The listing builds one solid part. Answer for the finished solid, in the listing's coordinates (mm). A direction names the side the tool comes from. Coordinates: 2 decimals unless noted, no trailing zeros. Write each loop counter-clockwise with the first axis right and the second up, starting at its lowest first coordinate (ties: lowest second). Pieces come first, ordered by that corner, then holes. Notation, with made-up numbers: M -28,52 L -18,52 A27 cw -18,73 Z; hole C -6,-7 d7. An arc over 180 degrees is marked long. Put each result on its own line as item: value. Start each with the question number.
```python
from build123d import *

# Parameters (mm, degrees)
BOSS_EXTRUDE1_DEPTH       = 25.4
F_4_0MM_DOWEL_HOLE1_D     = 4
F_4_0MM_DOWEL_HOLE1_DEPTH = 3.175
CUT_EXTRUDE1_REACH        = 51.202
SKETCH7_R                 = 5.08
SKETCH7_R_2               = 1.143
FILLET1_R                 = 3.175


with BuildPart() as part:
    # Sketch1 → Boss-Extrude1 (new body)
    with BuildSketch(Plane.XY):
        Polygon((-17.059275079, -16.268900152), (-29.759275079, -16.268900152), (-29.759275079, -36.588900152), (36.915724921, -36.588900152), (36.915724921, -33.413900152), (-26.584275079, -33.413900152), (-26.584275079, -19.443900152), (-17.059275079, -19.443900152), align=None)
    extrude(amount=BOSS_EXTRUDE1_DEPTH)

    # Ø4.0mm Dowel Hole1
    with Locations(Plane(origin=(0, -16.268900152, 0), x_dir=(1, 0, 0), z_dir=(0, 1, 0))):
        with Locations((-21.821775079, -7.9375), (-21.821775079, -17.4625)):
            Hole(F_4_0MM_DOWEL_HOLE1_D / 2, depth=F_4_0MM_DOWEL_HOLE1_DEPTH)

    # Sketch7 → Cut-Extrude1 (cut, up to next)
    with BuildSketch(Plane.XZ.offset(36.588900152), mode=Mode.PRIVATE) as cut_extrude1_sk1:
        with Locations(Location((23.199724921, 12.7, 0), (0, 0, 270))):
            Circle(SKETCH7_R)
    cut_extrude1_tool1 = extrude(cut_extrude1_sk1.sketch, amount=-CUT_EXTRUDE1_REACH, mode=Mode.PRIVATE) & part.part
    # Sketch7 → Cut-Extrude1 (cut, up to next)
    with BuildSketch(Plane.XZ.offset(36.588900152), mode=Mode.PRIVATE) as cut_extrude1_sk2:
        with Locations(Location((23.199724921, 5.2578, 0), (0, 0, 270))):
            Circle(SKETCH7_R_2)
    cut_extrude1_tool2 = extrude(cut_extrude1_sk2.sketch, amount=-CUT_EXTRUDE1_REACH, mode=Mode.PRIVATE) & part.part
    # Sketch7 → Cut-Extrude1 (cut, up to next)
    with BuildSketch(Plane.XZ.offset(36.588900152), mode=Mode.PRIVATE) as cut_extrude1_sk3:
        with Locations(Location((23.199724921, 20.1422, 0), (0, 0, 270))):
            Circle(SKETCH7_R_2)
    cut_extrude1_tool3 = extrude(cut_extrude1_sk3.sketch, amount=-CUT_EXTRUDE1_REACH, mode=Mode.PRIVATE) & part.part
    add(cut_extrude1_tool1.solids().sort_by_distance((23.199725, -36.5889, 12.7))[0], mode=Mode.SUBTRACT)
    add(cut_extrude1_tool2.solids().sort_by_distance((23.199725, -36.5889, 5.2578))[0], mode=Mode.SUBTRACT)
    add(cut_extrude1_tool3.solids().sort_by_distance((23.199725, -36.5889, 20.1422))[0], mode=Mode.SUBTRACT)

    # Fillet1
    fillet1_edges = [part.edges().sort_by_distance(p)[0] for p in [
        (-26.584275079, -33.413900152, 12.7),
        (-29.759275079, -36.588900152, 12.7),
        (-29.759275079, -16.268900152, 12.7),
    ]]
    fillet(fillet1_edges, radius=FILLET1_R)


solid = part.part
```
1) Straight lines are drawn through the part: probe 1 along Y at (x, z) = (-19.5, 9.25); probe 2 along Y at (x, z) = (-7, 9.25); probe 3 along Z at (x, y) = (-21, -18.25). For each, find the intervals that lie inside material, in ascending order.
2) For faces 4 (the face through (-26.584, -25, 13)), 5 (the face through (-17.059, -18, 13)), 6 (the face through (-20.235, -17.879, 18.679)), determine the directions among +Z, -Z, +X, -X, +Y, -Y from which every point of the face is accessible in a straight line to the end or side of a thin tool.
3) A cutting plane is placed at C-C on x = 2.5. Write down the section's boundary in (y, z), then the cut area to 3 significant figures.
4) Given pin 1 Ø10 at (y, z) = (-26.5, 14) entering from +X; pin 2 Ø1.5 at (y, z) = (-19, 5.5) entering from +X; pin 3 Ø5.5 at (y, z) = (-26.5, 17) entering from +X, each flat-ended and moving along its own axis, determine where each tip first touches the part or whether it passes through.
5) A cutting plane is placed at A-A on z = 12.7. Write down the section's boundary in (x, y) (3 decimals).
6) A cutting plane is placed at D-D on y = -24.5. Write down the section's boundary in (x, z), then the cut area to 3 significant figures.
7) A cutting plane is placed at B-B on z = 20.5. Write down the section's boundary in (x, y) (3 decimals), then the cut area to 3 significant figures.
8) Determine the mould class of faces 1 (the face through (-4, -34, 0)), 2 (the face through (24.333, -35.024, 5.407)), 3 (the face through (-28.8, -17.17, 12.88)) for opening direction Z: +Z half, -Z half, draft (parallel to the pull), parting line (faces both ways), or undercut.
Answers follow:
1. probe 1: y = -36.59 to -33.41, -19.44 to -16.27
1. probe 2: y = -36.59 to -33.41
1. probe 3: z = 0 to 6.11, 9.76 to 15.64, 19.29 to 25.4
2. face 4: +Z, -Z, +X
2. face 5: +Z, -Z, +X, +Y
2. face 6: +Y
3. outline: M -36.59,0 L -33.41,0 L -33.41,25.4 L -36.59,25.4 Z
3. area: 80.6 mm²
4. pin 1: stops at x = -26.32
4. pin 2: stops at x = -17.06
4. pin 3: stops at x = -26.58
5. outline: M -29.759,-33.414 A3.175 ccw -26.584,-36.589 L 18.12,-36.589 L 18.12,-33.414 L -23.409,-33.414 A3.175 cw -26.584,-30.239 L -26.584,-19.444 L -17.059,-19.444 L -17.059,-16.269 L -26.584,-16.269 A3.175 ccw -29.759,-19.444 Z; M 28.28,-36.589 L 36.916,-36.589 L 36.916,-33.414 L 28.28,-33.414 Z
6. outline: M -29.76,0 L -26.58,0 L -26.58,25.4 L -29.76,25.4 Z
6. area: 80.6 mm²
7. outline: M -29.759,-33.414 A3.175 ccw -26.584,-36.589 L 22.114,-36.589 L 22.114,-33.414 L -23.409,-33.414 A3.175 cw -26.584,-30.239 L -26.584,-19.444 L -17.059,-19.444 L -17.059,-16.269 L -26.584,-16.269 A3.175 ccw -29.759,-19.444 Z; M 24.285,-36.589 L 36.916,-36.589 L 36.916,-33.414 L 24.285,-33.414 Z
7. area: 287 mm²
8. face 1: -Z half
8. face 2: undercut
8. face 3: draft
